```python
from build123d import *

# Parameters (mm, degrees)
SKETCH1_W           = 190
SKETCH1_H           = 180
BOSS_EXTRUDE1_DEPTH = 4.7625


with BuildPart() as part:
    # Sketch1 → Boss-Extrude1 (new body)
    with BuildSketch(Plane(origin=(0, 0, 0), x_dir=(1, 0, 0), z_dir=(0, 1, 0))):
        Rectangle(SKETCH1_W, SKETCH1_H)
        with BuildLine():
            ThreePointArc((79.84375, 4.997557997), (-80, 0), (79.84375, -4.997557997))
            ThreePointArc((79.84375, -4.997557997), (85, 0), (79.84375, 4.997557997))
        make_face(mode=Mode.SUBTRACT)
    extrude(amount=BOSS_EXTRUDE1_DEPTH)


solid = part.part
```
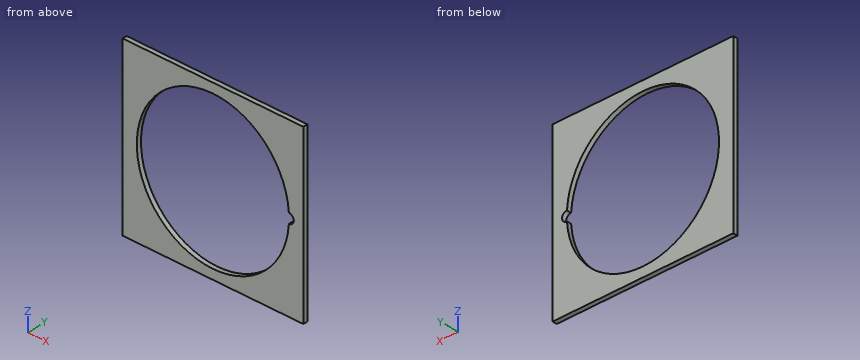
Design review of the part built by this model. Coordinates are the model's own, in mm. Round coordinates to 2 decimals unless told otherwise and drop trailing zeros. Order: outer loops, then holes, each group sorted by start corner. A loop starts at its lowest first (then second) coordinate and runs counter-clockwise, first axis right, second up. Notation, with made-up numbers: (-1.5, -10.5) - (24.5, -10.5) arc R14 cw to (24.5, -2.5) - close; hole circle Ø4 at (41.25, -39.5). An arc over 180 degrees is marked (long way). One line per question, with ' | ' between items.
Item 1: Take a section at A-A, the plane x = 0. Write out the cut boundary in (y, z), then the cut area to 4 significant figures.
Checks:
outline: (0, -90) - (4.76, -90) - (4.76, -80) - (0, -80) - close; (0, 80) - (4.76, 80) - (4.76, 90) - (0, 90) - close | area: 95.25 mm²
Item 2: Wall thickness on line 1 (Z direction, x = 0, y = 2.1); line 2 (Z direction, x = -71.5, y = 1.1); line 3 (X direction, y = 1, z = 23.5): over which ranges is each line inside the solid? List them lowest first. Write a range as [from, to].
Checks:
line 1: [-90, -80], [80, 90] | line 2: [-90, -35.89], [35.89, 90] | line 3: [-95, -76.47], [76.47, 95]
Item 3: Take a section at C-C, the plane y = 3.95. Write out the cut boundary in (x, z), then the cut area to 3 significant figures.
Checks:
outline: (-95, -90) - (95, -90) - (95, 90) - (-95, 90) - close; hole (79.84, -5) arc R5 ccw (long way) to (79.84, 5) arc R80 ccw (long way) to start | area: 14,100 mm²
Item 4: Take a section at B-B, the plane z = 0. Write out the cut boundary in (x, y).
Checks:
outline: (-95, 0) - (-80, 0) - (-80, 4.76) - (-95, 4.76) - close; (85, 0) - (95, 0) - (95, 4.76) - (85, 4.76) - close
